Verification items for the finished model (mm, model axes). Coordinates: 2 decimals unless noted, no trailing zeros. Order: outer loops, then holes, each group sorted by start corner. A loop starts at its lowest first (then second) coordinate and runs counter-clockwise, first axis right, second up. Notation, with made-up numbers: M -36,10.5 L -23,10.5 A18 ccw -23,17.5 Z; hole C -20.75,34.25 d5. An arc over 180 degrees is marked long. Return JSON: item names as keys, results as strings. Group by question number.
1. Gauge pin test, flat ends, axial feed: pin 1 (1 mm diameter, centred on x = 171.5, y = 0.5, fed in from -Z); pin 2 (8 mm diameter, centred on x = 232.5, z = -111.5, fed in from +Y); pin 3 (4 mm diameter, centred on x = 142, z = -220, fed in from +Y); pin 4 (1 mm diameter, centred on x = 233.5, z = -67, fed in from +Y). Record the tip position at first contact, or that the pin passes through.
2. Section check A-A, the plane x = 335.5. Record the cut outline in (y, z).
3. Section check B-B, the plane x = 214. Record the cut outline in (y, z), plus the area to 3 significant figures.
4. Material ranges on line 1 along Y through (x, z) = (294.5, -224); line 2 along Y through (x, z) = (230, -198), recorded low to high.
```python
from build123d import *

# Parameters (mm, degrees)
BOSS_EXTRUDE1_DEPTH = 250


with BuildPart() as part:
    # Sketch1 → Boss-Extrude1 (new body)
    with BuildSketch(Plane.XY):
        with BuildLine():
            Line((0, 0.079324087), (0, -10))
            Line((0, -10), (400, -10))
            Line((400, -10), (400, 0.079324087))
            ThreePointArc((400, 0.079324087), (395, -1.974497919), (390, 0.079324087))
            ThreePointArc((390, 0.079324087), (385, 2.133146093), (380, 0.079324087))
            ThreePointArc((380, 0.079324087), (375, -1.974497919), (370, 0.079324087))
            ThreePointArc((370, 0.079324087), (365, 2.133146093), (360, 0.079324087))
            ThreePointArc((360, 0.079324087), (355, -1.974497919), (350, 0.079324087))
            ThreePointArc((350, 0.079324087), (345, 2.133146093), (340, 0.079324087))
            ThreePointArc((340, 0.079324087), (335, -1.974497919), (330, 0.079324087))
            ThreePointArc((330, 0.079324087), (325, 2.133146093), (320, 0.079324087))
            ThreePointArc((320, 0.079324087), (315, -1.974497919), (310, 0.079324087))
            ThreePointArc((310, 0.079324087), (305, 2.133146093), (300, 0.079324087))
            ThreePointArc((300, 0.079324087), (295, -1.974497919), (290, 0.079324087))
            ThreePointArc((290, 0.079324087), (285, 2.133146093), (280, 0.079324087))
            ThreePointArc((280, 0.079324087), (275, -1.974497919), (270, 0.079324087))
            ThreePointArc((270, 0.079324087), (265, 2.133146093), (260, 0.079324087))
            ThreePointArc((260, 0.079324087), (255, -1.974497919), (250, 0.079324087))
            ThreePointArc((250, 0.079324087), (245, 2.133146093), (240, 0.079324087))
            ThreePointArc((240, 0.079324087), (235, -1.974497919), (230, 0.079324087))
            ThreePointArc((230, 0.079324087), (225, 2.133146093), (220, 0.079324087))
            ThreePointArc((220, 0.079324087), (215, -1.974497919), (210, 0.079324087))
            ThreePointArc((210, 0.079324087), (205, 2.133146093), (200, 0.079324087))
            ThreePointArc((200, 0.079324087), (195, -1.974497919), (190, 0.079324087))
            ThreePointArc((190, 0.079324087), (185, 2.133146093), (180, 0.079324087))
            ThreePointArc((180, 0.079324087), (175, -1.974497919), (170, 0.079324087))
            ThreePointArc((170, 0.079324087), (165, 2.133146093), (160, 0.079324087))
            ThreePointArc((160, 0.079324087), (155, -1.974497919), (150, 0.079324087))
            ThreePointArc((150, 0.079324087), (145, 2.133146093), (140, 0.079324087))
            ThreePointArc((140, 0.079324087), (135, -1.974497919), (130, 0.079324087))
            ThreePointArc((130, 0.079324087), (125, 2.133146093), (120, 0.079324087))
            ThreePointArc((120, 0.079324087), (115, -1.974497919), (110, 0.079324087))
            ThreePointArc((110, 0.079324087), (105, 2.133146093), (100, 0.079324087))
            ThreePointArc((100, 0.079324087), (95, -1.974497919), (90, 0.079324087))
            ThreePointArc((90, 0.079324087), (85, 2.133146093), (80, 0.079324087))
            ThreePointArc((80, 0.079324087), (75, -1.974497919), (70, 0.079324087))
            ThreePointArc((70, 0.079324087), (65, 2.133146093), (60, 0.079324087))
            ThreePointArc((60, 0.079324087), (55, -1.974497919), (50, 0.079324087))
            ThreePointArc((50, 0.079324087), (45, 2.133146093), (40, 0.079324087))
            ThreePointArc((40, 0.079324087), (35, -1.974497919), (30, 0.079324087))
            ThreePointArc((30, 0.079324087), (25, 2.133146093), (20, 0.079324087))
            ThreePointArc((20, 0.079324087), (15, -1.974497919), (10, 0.079324087))
            ThreePointArc((10, 0.079324087), (5, 2.133146093), (0, 0.079324087))
        make_face()
    extrude(amount=-BOSS_EXTRUDE1_DEPTH)


solid = part.part
```
Answers follow:
{
 "1": {"pin 1": "through", "pin 2": "y = 1.21", "pin 3": "y = 2.06", "pin 4": "y = -1.69"},
 "2": {"outline": "M -10,-250 L -1.96,-250 L -1.96,0 L -10,0 Z"},
 "3": {"outline": "M -10,-250 L -1.9,-250 L -1.9,0 L -10,0 Z", "area": "2,020 mm^2"},
 "4": {"line 1": "-10 to -1.96", "line 2": "-10 to 0.08"}
}
